```python
from build123d import *

# Parameters (mm, degrees)
F0_R     = 10
F1_DEPTH = 22
F3_D     = 13
F3_DEPTH = 17
F3_TIP   = 3.9055940237
F5_DEPTH = 18
F6_DEPTH = 17


with BuildPart() as f1:
    # F0 (on Top) → F1 (new body)
    with BuildSketch(Plane.XY):
        Circle(F0_R)
    extrude(amount=F1_DEPTH)

    # F3
    with Locations(Plane(origin=(0, 0, 0), x_dir=(1, 0, 0), z_dir=(0, 0, -1))):
        with Locations((0, 0)):
            Hole(F3_D / 2, depth=F3_DEPTH)
            with Locations((0, 0, -(F3_DEPTH + F3_TIP / 2))):  # 118° drill point
                Cone(0, F3_D / 2, F3_TIP, mode=Mode.SUBTRACT)

    # F4 (on Top) → F5 (cut)
    with BuildSketch(Plane.XY):
        with BuildLine():
            Line((2.770723775, -9.6206208691), (2.770723775, -5.7840836234))
            ThreePointArc((2.770723775, -5.7840836234), (-4.5716731582, -4.4980371424), (-5.7383336819, 2.8642730588))
            Line((-5.7383336819, 2.8642730588), (-9.7194789065, 2.401038511))
            ThreePointArc((-9.7194789065, 2.401038511), (-6.9427208666, -7.2133129083), (2.770723775, -9.6206208691))
        make_face()
    extrude(amount=F5_DEPTH, mode=Mode.SUBTRACT)

    # F4 (on Top) → F6 (join)
    with BuildSketch(Plane.XY):
        with BuildLine():
            Line((2.770723775, -9.6206208691), (2.770723775, -5.7840836234))
            ThreePointArc((2.770723775, -5.7840836234), (-4.5716731582, -4.4980371424), (-5.7383336819, 2.8642730588))
            Line((-5.7383336819, 2.8642730588), (-9.7194789065, 2.401038511))
            ThreePointArc((-9.7194789065, 2.401038511), (-6.9427208666, -7.2133129083), (2.770723775, -9.6206208691))
        make_face()
    extrude(amount=F6_DEPTH)


solid = f1.part
```
The model under review builds one solid part; all positions refer to its coordinate system, in mm. A direction names the side the tool comes from. Round coordinates to 2 decimals unless told otherwise and drop trailing zeros. Loops run counter-clockwise (first coordinate to the right, second up) from the corner with the lowest first, then second, coordinate; pieces in that order, holes last. Notation, with made-up numbers: (-39.5, 49) -> (5.5, 49) arc R24 ccw to (5.5, 79) -> close; hole circle Ø11 at (72, -27). An arc over 180 degrees is marked (long way). Answer as a JSON object with one key per item and string values. Group by question number.
1) For line 1 (X direction, y = 0, z = 6); line 2 (Z direction, x = -4.5, y = -5), list the stretches that pass through material, from the lowest coordinate up. Write a range as [from, to].
2) We need section D-D on y = 8.25. Write out the cut boundary in (x, z), then the cut area to 3 significant figures.
3) Mouldability with a two-part tool opening along Z and no side actions: class faces 4 (the face through (2.771, -7.7, 17.5)), 5 (the face through (-7.05, -7.11, 8.38)), 6 (the face through (-4.49, -4.58, 17.52)), 7 (the face through (0, -7, 0)) as released by +Z, released by -Z, zero draft, split by the parting line, or undercut.
4) We need section B-B on y = -7. Write out the cut boundary in (x, z), then the cut area to 3 significant figures.
5) For pin 1 Ø8 at (y, z) = (5.5, 5) entering from +X; pin 2 Ø6 at (x, z) = (7.5, 9.5) entering from -Y; pin 3 Ø3 at (x, z) = (3, 12) entering from +Y, all flat-tipped, find the tip position at first contact; note any pin that passes through.
6) We need section C-C on x = -7.5. Write out the cut boundary in (y, z).
7) For faces 1 (the face through (-4.49, -4.58, 8.38)), 2 (the face through (0, 0, 22)), 3 (the face through (-7.695, 2.637, 17.493)), list the 3-axis set-ups (+Z, -Z, +X, -X, +Y, -Y) from which the entire face can be reached by the end or side of a thin tool; tool diameter is ignored.
Result set:
{
 "1": {"line 1": "[-10.01, -6.41], [6.5, 10]", "line 2": "[0, 17], [18, 22]"},
 "2": {"outline": "(-5.65, 0) -> (5.65, 0) -> (5.65, 22) -> (-5.65, 22) -> close", "area": "249 mm²"},
 "3": {"face 4": "undercut", "face 5": "zero draft", "face 6": "undercut", "face 7": "released by -Z"},
 "4": {"outline": "(-7.16, 0) -> (7.14, 0) -> (7.14, 22) -> (-7.14, 22) -> (-7.14, 18) -> (2.77, 18) -> (2.77, 17) -> (-7.16, 17) -> close", "area": "305 mm²"},
 "5": {"pin 1": "x = 9.89", "pin 2": "y = -8.93", "pin 3": "y = 9.89"},
 "6": {"outline": "(-6.63, 0) -> (6.61, 0) -> (6.61, 22) -> (-6.61, 22) -> (-6.61, 18) -> (2.66, 18) -> (2.66, 17) -> (-6.63, 17) -> close"},
 "7": {"face 1": "-Z", "face 2": "+Z, +X, -X, +Y, -Y", "face 3": "none"}
}
